Verification items for the finished model (mm, model axes). Give positions to 0.01 mm unless a question says otherwise; leave off trailing zeros. Write each loop counter-clockwise with the first axis right and the second up, starting at its lowest first coordinate (ties: lowest second). Pieces come first, ordered by that corner, then holes.
from build123d import *

# Parameters (mm, degrees)
F0_R     = 71.12
F0_R_2   = 12.7
F0_R_3   = 6.35
F1_DEPTH = 6.35
F2_R     = 12.7
F2_R_2   = 6.35
F3_DEPTH = 25.4
F4_R     = 5.08


with BuildPart() as f1:
    # F0 (on Front) → F1 (new body)
    with BuildSketch(Plane.XZ):
        Circle(F0_R)
        with BuildLine():
            Line((-6.839159, -17.78), (-6.839159, -63.130626))
            ThreePointArc((-6.839159, -63.130626), (-44.901281, -44.901281), (-63.130626, -6.839159))
            Line((-63.130626, -6.839159), (-17.78, -6.839159))
            ThreePointArc((-17.78, -6.839159), (-13.470384, -13.470384), (-6.839159, -17.78))
        make_face(mode=Mode.SUBTRACT)
        Circle(F0_R_2, mode=Mode.SUBTRACT)
        with BuildLine():
            Line((17.78, -6.839159), (63.130626, -6.839159))
            ThreePointArc((63.130626, -6.839159), (44.901281, -44.901281), (6.839159, -63.130626))
            Line((6.839159, -63.130626), (6.839159, -17.78))
            ThreePointArc((6.839159, -17.78), (13.470384, -13.470384), (17.78, -6.839159))
        make_face(mode=Mode.SUBTRACT)
        with BuildLine():
            Line((-6.839159, 63.130626), (-6.839159, 17.78))
            ThreePointArc((-6.839159, 17.78), (-13.470384, 13.470384), (-17.78, 6.839159))
            Line((-17.78, 6.839159), (-63.130626, 6.839159))
            ThreePointArc((-63.130626, 6.839159), (-44.901281, 44.901281), (-6.839159, 63.130626))
        make_face(mode=Mode.SUBTRACT)
        with BuildLine():
            ThreePointArc((6.839159, 63.130626), (44.901281, 44.901281), (63.130626, 6.839159))
            Line((63.130626, 6.839159), (17.78, 6.839159))
            ThreePointArc((17.78, 6.839159), (13.470384, 13.470384), (6.839159, 17.78))
            Line((6.839159, 17.78), (6.839159, 63.130626))
        make_face(mode=Mode.SUBTRACT)
        Circle(F0_R_2)
        Circle(F0_R_3, mode=Mode.SUBTRACT)
    extrude(amount=F1_DEPTH)

    # F2 (on face) → F3 (join)
    with BuildSketch(Plane.XZ.offset(6.35)):
        Circle(F2_R)
        Circle(F2_R_2, mode=Mode.SUBTRACT)
    extrude(amount=F3_DEPTH)

    # F4
    f4_edges = [f1.edges().sort_by_distance(p)[0] for p in [
        (6.839159, -3.175, 63.130626),
        (6.839159, -3.175, 17.78),
        (17.78, -3.175, 6.839159),
        (63.130626, -3.175, 6.839159),
        (17.78, -3.175, -6.839159),
        (6.839159, -3.175, -17.78),
        (63.130626, -3.175, -6.839159),
        (6.839159, -3.175, -63.130626),
        (-6.839159, -3.175, -63.130626),
        (-17.78, -3.175, -6.839159),
        (-6.839159, -3.175, -17.78),
        (-63.130626, -3.175, -6.839159),
        (-17.78, -3.175, 6.839159),
        (-63.130626, -3.175, 6.839159),
        (-6.839159, -3.175, 63.130626),
        (-6.839159, -3.175, 17.78),
    ]]
    fillet(f4_edges, radius=F4_R)


solid = f1.part
Item 1: Scan lines: line 1 along Z through (x, y) = (0, -17); line 2 along Z through (x, y) = (23.5, -2.5); line 3 along X through (y, z) = (-6, 32.5). Record each from-to range of solid material in increasing order.
Answer key:
line 1: z = -12.7 to -6.35, 6.35 to 12.7
line 2: z = -67.13 to -58.99, -6.84 to 6.84, 58.99 to 67.13
line 3: x = -63.26 to -54.55, -6.84 to 6.84, 54.55 to 63.26
Item 2: Depth check by flat-ended pin: pin 1 (1.9 mm diameter, centred on y = -3.5, z = 32.5, fed in from -X); pin 2 (1.5 mm diameter, centred on x = -4, y = -16.5, fed in from +Z); pin 3 (1.9 mm diameter, centred on y = -3, z = 30.5, fed in from +X). Enter the tip coordinate at first touch or a pass-through.
Answer key:
pin 1: stops at x = -63.74
pin 2: stops at z = 12.28
pin 3: stops at x = 64.69
Item 3: Sectioned sample at B-B on z = 0. Record the cut outline in (x, y), then the cut area to 3 significant figures.
Answer key:
outline: (-71.12, -6.35) - (-12.7, -6.35) - (-12.7, -31.75) - (-6.35, -31.75) - (-6.35, 0) - (-71.12, 0) - close; (6.35, -31.75) - (12.7, -31.75) - (12.7, -6.35) - (71.12, -6.35) - (71.12, 0) - (6.35, 0) - close
area: 1,150 mm2
Item 4: Sectioned sample at A-A on y = -3. State how many separate pieces and enclosed holes the cut face has, then the cut area to 3 significant figures.
Answer key:
separate pieces: 1
enclosed holes: 5
area: 6,760 mm2
Item 5: Sectioned sample at D-D on x = -25.5. Record the cut outline in (y, z), then the cut area to 3 significant figures.
Answer key:
outline: (-6.35, -66.39) - (0, -66.39) - (0, -58.15) - (-6.35, -58.15) - close; (-6.35, -6.84) - (0, -6.84) - (0, 6.84) - (-6.35, 6.84) - close; (-6.35, 58.15) - (0, 58.15) - (0, 66.39) - (-6.35, 66.39) - close
area: 191 mm2
Item 6: Sectioned sample at C-C on x = 0. Record the cut outline in (y, z), then the cut area to 3 significant figures.
Answer key:
outline: (-31.75, -12.7) - (-6.35, -12.7) - (-6.35, -71.12) - (0, -71.12) - (0, -6.35) - (-31.75, -6.35) - close; (-31.75, 6.35) - (0, 6.35) - (0, 71.12) - (-6.35, 71.12) - (-6.35, 12.7) - (-31.75, 12.7) - close
area: 1,150 mm2
Item 7: Release check for a two-part mould opening along X. For faces 1 (the face through (-2.75, -18.87, -12.4)), 2 (the face through (-1, 0, -15)), 3 (the face through (18.46, -3.22, 7.51)), 4 (the face through (-8.666, -3.219, 61.093)) record: released by +X, released by -X, zero draft, split by the parting line, or undercut.
Answer key:
face 1: split by the parting line
face 2: zero draft
face 3: undercut
face 4: undercut
